from build123d import *

# Parameters (mm, degrees)
SKETCH1_W           = 72
SKETCH1_H           = 35
BOSS_EXTRUDE1_DEPTH = 10
FILLET1_R           = 12
SKETCH3_W           = 5
SKETCH3_H           = 4
CUT_EXTRUDE1_DEPTH  = 89
SKETCH6_R           = 6
BOSS_EXTRUDE2_DEPTH = 10
FILLET2_R           = 15
M12_TAPPED_HOLE1_D  = 10.2
SKETCH11_R          = 15
BOSS_EXTRUDE5_DEPTH = 5
SKETCH18_R          = 6
CUT_EXTRUDE2_DEPTH  = 91.255193756
RIB1_REACH          = 87.013
SKETCH19_WALL_W     = 212.026468528
SKETCH19_WALL_H     = 10


with BuildPart() as part:
    # Sketch1 → Boss-Extrude1 (new body)
    with BuildSketch(Plane(origin=(0, 0, 0), x_dir=(1, 0, 0), z_dir=(0, 1, 0))):
        Rectangle(SKETCH1_W, SKETCH1_H)
    extrude(amount=BOSS_EXTRUDE1_DEPTH)

    # Fillet1
    fillet1_edges = [part.edges().sort_by_distance(p)[0] for p in [
        (36, 5, 17.5),
        (-36, 5, 17.5),
    ]]
    fillet(fillet1_edges, radius=FILLET1_R)

    # Sketch3 → Cut-Extrude1 (cut)
    with BuildSketch(Plane(origin=(36, 0, 0), x_dir=(0, 0, -1), z_dir=(1, 0, 0))):
        with Locations((15, 8)):
            Rectangle(SKETCH3_W, SKETCH3_H)
    extrude(amount=-CUT_EXTRUDE1_DEPTH, mode=Mode.SUBTRACT)

    # Sketch6 → Boss-Extrude2 (add)
    with BuildSketch(Plane(origin=(0, 0, -12.5), x_dir=(-1, 0, 0), z_dir=(0, 0, -1))):
        with BuildLine():
            Line((14.970991041, 10), (-15, 10))
            Line((-15, 10), (-15, 60))
            ThreePointArc((-15, 60), (-0.466440987, 74.992746006), (14.970991041, 60.932430832))
            Line((14.970991041, 60.932430832), (14.970991041, 10))
        make_face()
        with Locations((0, 60)):
            Circle(SKETCH6_R, mode=Mode.SUBTRACT)
    extrude(amount=-BOSS_EXTRUDE2_DEPTH)

    # Fillet2
    fillet2_edges = [part.edges().sort_by_distance(p)[0] for p in [
        (-14.970991041, 10, -7.5),
        (15, 10, -7.5),
    ]]
    fillet(fillet2_edges, radius=FILLET2_R)

    # M12 Tapped Hole1 (through all)
    with Locations(Plane(origin=(0, 10, 0), x_dir=(1, 0, 0), z_dir=(0, 1, 0))):
        with Locations((24, -5.5), (-24, -5.5)):
            Hole(M12_TAPPED_HOLE1_D / 2)

    # Sketch11 → Boss-Extrude5 (add)
    with BuildSketch(Plane(origin=(0, 0, -12.5), x_dir=(-1, 0, 0), z_dir=(0, 0, -1))):
        with Locations((0, 60)):
            Circle(SKETCH11_R)
    extrude(amount=BOSS_EXTRUDE5_DEPTH)

    # Sketch18 → Cut-Extrude2 (cut, through all)
    with BuildSketch(Plane(origin=(0, 0, -17.5), x_dir=(-1, 0, 0), z_dir=(0, 0, -1))):
        with Locations((0, 60)):
            Circle(SKETCH18_R)
    extrude(amount=-CUT_EXTRUDE2_DEPTH, mode=Mode.SUBTRACT)

    # Sketch19 wall → Rib1 (add, up to next)
    with BuildSketch(Plane(origin=(0, 27.320508076, 7.5), x_dir=(0, 0.866025403782, -0.500000000004), z_dir=(0, 0.500000000004, 0.866025403782)), mode=Mode.PRIVATE) as rib1_sk1:
        Rectangle(SKETCH19_WALL_W, SKETCH19_WALL_H)
    rib1_tool1 = extrude(rib1_sk1.sketch, amount=-RIB1_REACH, mode=Mode.PRIVATE) - part.part
    add(rib1_tool1.solids().sort_by_distance((0, 27.320508076, 7.5))[0])


solid = part.part
Design review of the part built by this model. Coordinates are the model's own, in mm. A direction names the side the tool comes from. Give positions to 0.01 mm unless a question says otherwise; leave off trailing zeros. Order: outer loops, then holes, each group sorted by start corner. A loop starts at its lowest first (then second) coordinate and runs counter-clockwise, first axis right, second up. Notation, with made-up numbers: (71.5, 70.5) - (115.5, 70.5) arc R22 ccw to (115.5, 88.5) - close; hole circle Ø8 at (62.25, 89.5). An arc over 180 degrees is marked (long way). Write item = value, one per line. Start each with the question number.
Q1. We need section D-D on x = -20.5. State the section outline as (y, z) points.
Q2. Mouldability with a two-part tool opening along X and no side actions: class faces 6 (the face through (-18.905, 4.93, 5.276)), 7 (the face through (-36, 5, -6)), 8 (the face through (5, 21, 6)) as released by +X, released by -X, zero draft, split by the parting line, or undercut.
Q3. Clearance check with flat-ended pins moving along their axes: pin 1 Ø3 at (x, z) = (15.5, 0.5) entering from +Y; pin 2 Ø5 at (x, z) = (-12, -10.5) entering from +Y; pin 3 Ø5.5 at (x, z) = (10.5, -14) entering from +Y. State where each tip first meets the part, or that it passes through.
Q4. To check wall thickness, follow L1, parallel to Z at x = 24, y = 3; L2, parallel to Y at x = 0, z = -5; L3, parallel to X at y = 5, z = 5. State the ranges of each line that lie inside material, in increasing order. Write a range as from..to.
Q5. We need section A-A on x = 0. State the section outline as (y, z) points, plus the area to 3 significant figures.
Q6. Tool access review of faces 1 (the face through (17, 10, 6)), 2 (the face through (15, 42, -8)), 3 (the face through (1, 6, -15)), 4 (the face through (-5, 21, 6)), 5 (the face through (6, 43, -2.5)): name each direction out of +Z, -Z, +X, -X, +Y, -Y from which nothing blocks a thin tool from reaching the whole face with its end or side.
Q7. We need section B-B on z = 13. State the section outline as (x, y) points, plus the area to 3 significant figures.
Q8. We need section C-C on y = 50.5. State the section outline as (x, z) points.
Working result:
q1.outline = (0, -17.5) - (6, -17.5) - (6, -12.5) - (13.37, -12.5) - (13.37, -2.5) - (10, -2.5) - (10, 1.79) - (0, 1.79) - close; (0, 9.21) - (10, 9.21) - (10, 17.5) - (0, 17.5) - close
q2.face_6 = undercut
q2.face_7 = released by -X
q2.face_8 = released by +X
q3.pin_1 = 10
q3.pin_2 = 71.61
q3.pin_3 = 72.84
q4.L1 = -17.5..0.4, 10.6..17.5
q4.L2 = 0..54, 66..75
q4.L3 = -36..-29.08, -18.92..18.92, 29.08..36
q5.outline = (0, -17.5) - (6, -17.5) - (6, -12.5) - (45, -12.5) - (45, -17.5) - (54, -17.5) - (54, -2.5) - (44.64, -2.5) - (10, 17.5) - (0, 17.5) - close; (66, -17.5) - (75, -17.5) - (75, -2.5) - (66, -2.5) - close
q5.area = 1,300 mm²
q6.face_1 = +Z, +X, +Y
q6.face_2 = +Z, -Z, +X, +Y
q6.face_3 = -Z, +X, -X
q6.face_4 = +Z, -X, +Y
q6.face_5 = +Z, +Y
q7.outline = (-33.37, 0) - (33.37, 0) - (33.37, 10) - (5, 10) - (5, 17.79) - (-5, 17.79) - (-5, 10) - (-33.37, 10) - close
q7.area = 745 mm²
q8.outline = (-14.97, -12.5) - (-11.61, -12.5) - (-11.61, -17.5) - (11.61, -17.5) - (11.61, -12.5) - (15, -12.5) - (15, -2.5) - (-14.97, -2.5) - close
